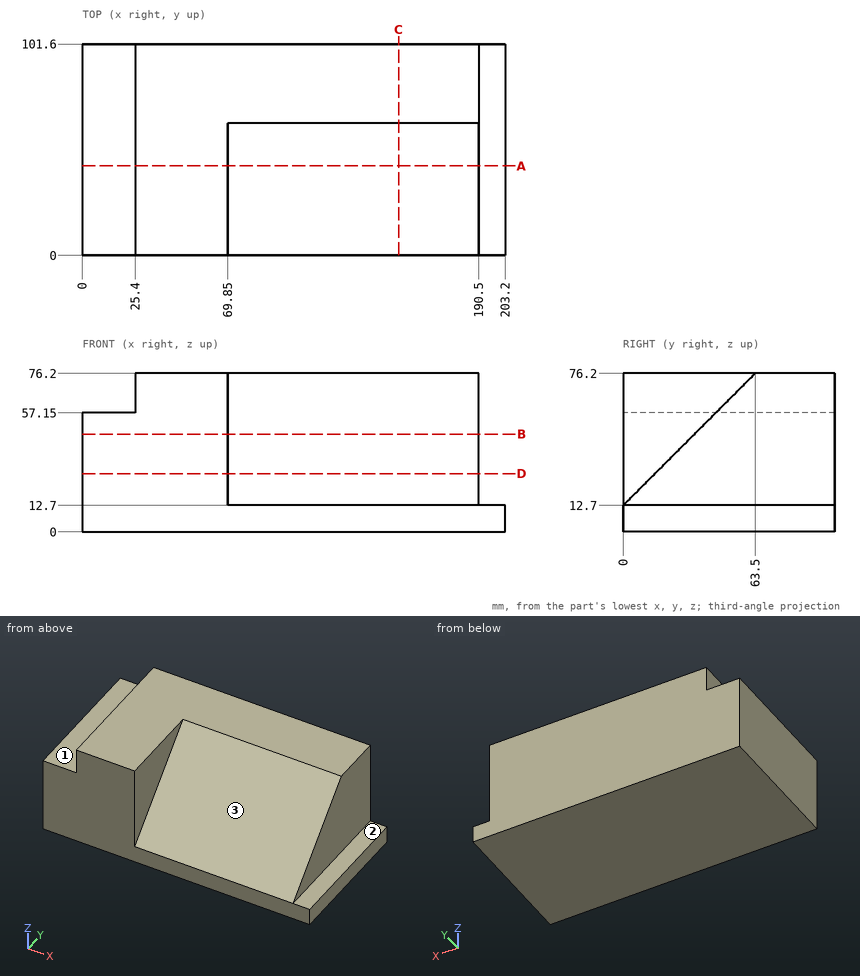
Answer from the drawing. Dimensions are ordinates in mm from the lowest x, y and z of the part. A direction names the side the tool comes from. Give positions to 0.01 mm unless a question says otherwise; leave off trailing zeros. Write each loop counter-clockwise with the first axis right and the second up, starting at its lowest first coordinate (ties: lowest second). Pieces come first, ordered by that corner, then holes.
1) A tool of negligible diameter and unlimited length cuts with its end or side. For the marked faces 1, 2 and 3, from which of +Z, -Z, +X, -X, +Y, -Y can it reach the whole face along a straight path? Write none if from no direction.
2) Given P1, Ø6.5, axis at x = 196.5, y = 50.5, coming from the +Z side; P2, Ø12.5, axis at x = 11.5, y = 37.5, coming from the +Z side; P3, Ø19, axis at y = 36.5, z = 40.5, coming from the +X side, each flat-ended and moving along its own axis, determine where each tip first touches the part or whether it passes through.
3) Section C-C (x = 152) is taken. Write down the section's boundary in (y, z), and give its area (3 significant figures).
4) Section D-D (z = 28) is taken. Write down the section's boundary in (x, y).
5) Section A-A (y = 43) is taken. Write down the section's boundary in (x, z), and give its area (3 significant figures).
6) Find the intervals of material crossed by L1, parallel to X at y = 54.5, z = 20.5; L2, parallel to Z at x = 15, y = 92.5; L3, parallel to X at y = 67.5, z = 69, in increasing order.
7) Section B-B (z = 47) is taken. Write down the section's boundary in (x, y).
Response:
1. face 1: +Z, -X, +Y, -Y
1. face 2: +Z, +X, +Y, -Y
1. face 3: +Z, +X, -Y
2. P1: stops at z = 12.7
2. P2: stops at z = 57.15
2. P3: stops at x = 190.5
3. outline: (0, 0) - (101.6, 0) - (101.6, 76.2) - (63.5, 76.2) - (0, 12.7) - close
3. area: 5,730 mm2
4. outline: (0, 0) - (69.85, 0) - (69.85, 15.3) - (190.5, 15.3) - (190.5, 101.6) - (0, 101.6) - close
5. outline: (0, 0) - (203.2, 0) - (203.2, 12.7) - (190.5, 12.7) - (190.5, 55.7) - (69.85, 55.7) - (69.85, 76.2) - (25.4, 76.2) - (25.4, 57.15) - (0, 57.15) - close
5. area: 11,700 mm2
6. L1: x = 0 to 190.5
6. L2: z = 0 to 57.15
6. L3: x = 25.4 to 190.5
7. outline: (0, 0) - (69.85, 0) - (69.85, 34.3) - (190.5, 34.3) - (190.5, 101.6) - (0, 101.6) - close
